Verification items for the finished model (mm, model axes). A direction names the side the tool comes from. Round coordinates to 2 decimals unless told otherwise and drop trailing zeros. Order: outer loops, then holes, each group sorted by start corner. A loop starts at its lowest first (then second) coordinate and runs counter-clockwise, first axis right, second up. Notation, with made-up numbers: (39, 49) -> (57, 49) arc R14 ccw to (57, 67) -> close; hole circle Ø10 at (-1.75, -9.5). An arc over 180 degrees is marked (long way). Put each result on its own line as item: value.
from build123d import *

# Parameters (mm, degrees)
SKETCH051_R             = 12.5
PAD018_DEPTH            = 13
SKETCH055_R             = 2.5
POCKET030_DEPTH         = 8
SKETCH056_R             = 2.5
POCKET029_DEPTH         = 8
BODY013_PLACEMENT_ANGLE = -90


with BuildPart() as part:
    # Sketch051 → Pad018 (new body, symmetric)
    with BuildSketch(Plane.XZ):
        Circle(SKETCH051_R)
    extrude(amount=PAD018_DEPTH, both=True)

    # Sketch055 (on Face3 of Pad018) → Pocket030 (cut)
    with BuildSketch(Plane.XZ.offset(13)):
        Circle(SKETCH055_R)
    extrude(amount=-POCKET030_DEPTH, mode=Mode.SUBTRACT)

    # Sketch056 (on Face2 of Pocket030) → Pocket029 (cut)
    with BuildSketch(Plane(origin=(0, 13, 0), x_dir=(1, 0, 0), z_dir=(0, 1, 0))):
        Circle(SKETCH056_R)
    extrude(amount=-POCKET029_DEPTH, mode=Mode.SUBTRACT)


with BuildPart() as part_1:
    # Body013 placement: moved
    add(part.part.moved(Location((-17.75, 0, 150))).rotate(Axis((-17.75, 0, 150), (0, 0, 1)), BODY013_PLACEMENT_ANGLE))


solid = part_1.part
Item 1: Gauge pin test, flat ends, axial feed: pin 1 Ø10 at (x, y) = (-17.5, 6.5) entering from -Z; pin 2 Ø2 at (x, z) = (-24, 141) entering from +Y; pin 3 Ø3 at (x, z) = (-11, 140.5) entering from -Y. Record the tip position at first contact, or that the pin passes through.
Check sheet entries:
pin 1: stops at z = 137.59
pin 2: stops at y = 9.6
pin 3: stops at y = -9.6
Item 2: Release check for a two-part mould opening along Z. For faces 4 (the cylindrical face through (-17.932, 1.627, 162.394)), 5 (the flat face through (-4.75, 0, 147)), 6 (the flat face through (-12.75, 0, 150)), 7 (the flat face through (-22.75, 0, 150)) record: +Z half, -Z half, draft (parallel to the pull), parting line (faces both ways), or undercut.
Check sheet entries:
face 4: parting line
face 5: draft
face 6: undercut
face 7: undercut
Item 3: Section check C-C on y = 0. Record the boundary of the cut face in (x, z), then the cut area to 3 significant figures.
Check sheet entries:
outline: (-30.75, 137.5) -> (-4.75, 137.5) -> (-4.75, 147.5) -> (-12.75, 147.5) -> (-12.75, 152.5) -> (-4.75, 152.5) -> (-4.75, 162.5) -> (-30.75, 162.5) -> (-30.75, 152.5) -> (-22.75, 152.5) -> (-22.75, 147.5) -> (-30.75, 147.5) -> close
area: 570 mm^2
Item 4: Section check D-D on x = -19.75. Record the boundary of the cut face in (y, z), then the cut area to 3 significant figures.
Check sheet entries:
outline: circle Ø25 at (0, 150)
area: 491 mm^2
Item 5: Section check A-A on z = 150. Record the boundary of the cut face in (x, y), then the cut area to 3 significant figures.
Check sheet entries:
outline: (-30.75, -12.5) -> (-4.75, -12.5) -> (-4.75, -2.5) -> (-12.75, -2.5) -> (-12.75, 2.5) -> (-4.75, 2.5) -> (-4.75, 12.5) -> (-30.75, 12.5) -> (-30.75, 2.5) -> (-22.75, 2.5) -> (-22.75, -2.5) -> (-30.75, -2.5) -> close
area: 570 mm^2
Item 6: Material ranges on L1, parallel to Z at x = -26, y = 0; L2, parallel to Y at x = -6.5, z = 151.5; L3, parallel to X at y = 1.5, z = 151.75, recorded low to high. Write a range as [from, to].
Check sheet entries:
L1: z = [137.5, 147.5], [152.5, 162.5]
L2: y = [-12.41, -2], [2, 12.41]
L3: x = [-22.75, -12.75]
Item 7: Section check B-B on x = -28. Record the boundary of the cut face in (y, z), then the cut area to 3 significant figures.
Check sheet entries:
outline: circle Ø25 at (0, 150); hole circle Ø5 at (0, 150)
area: 471 mm^2
Item 8: Tool access check on faces 1 (the flat face through (-30.75, 0, 147)), 2 (the cylindrical face through (-26.81, 0.33, 152.48)), 3 (the cylindrical face through (-8.69, 0.33, 147.52)). Record the directions out of +Z, -Z, +X, -X, +Y, -Y that give a thin tool (end or side, any length) a straight path to the whole face; none if there is none.
Check sheet entries:
face 1: +Z, -Z, -X, +Y, -Y
face 2: -X
face 3: +X
